from build123d import *

# Parameters (mm, degrees)
SKETCH1_W                = 20
SKETCH1_H                = 8
SKETCH1_R                = 1.25
BOSS_EXTRUDE1_DEPTH      = 2
BOSS_EXTRUDE2_DEPTH      = 4
BOSS_EXTRUDE2_DEPTH_BACK = 2
SKETCH3_R                = 0.5
SKETCH3_R_2              = 1
SKETCH5_R                = 1.5875
CUT_EXTRUDE1_DEPTH       = 4
FILLET1_R                = 1


with BuildPart() as part:
    # Sketch1 → Boss-Extrude1 (new body)
    with BuildSketch(Plane(origin=(0, 0, 0), x_dir=(1, 0, 0), z_dir=(0, 1, 0))):
        with Locations((10, 4)):
            Rectangle(SKETCH1_W, SKETCH1_H)
        with Locations(Location((4, 4, 0), (0, 0, 270))):
            Circle(SKETCH1_R, mode=Mode.SUBTRACT)
        with Locations(Location((16, 4, 0), (0, 0, 270))):
            Circle(SKETCH1_R, mode=Mode.SUBTRACT)
    extrude(amount=BOSS_EXTRUDE1_DEPTH)

    # Sketch3 → Boss-Extrude2 (add, two sides: drawn at the far end of the back side and taken through both)
    with BuildSketch(Plane.XY.offset(-BOSS_EXTRUDE2_DEPTH_BACK)):
        with BuildLine():
            Line((5.825, 2), (5.825, 6))
            ThreePointArc((5.825, 6), (10, 10.175), (14.175, 6))
            Line((14.175, 6), (14.175, 2))
            Line((14.175, 2), (14.175, 0))
            Line((14.175, 0), (5.825, 0))
            Line((5.825, 0), (5.825, 2))
        make_face()
        with Locations((10, 8.4875)):
            Circle(SKETCH3_R, mode=Mode.SUBTRACT)
        with Locations((12.154238192, 4.75625)):
            Circle(SKETCH3_R, mode=Mode.SUBTRACT)
        with Locations((7.845761808, 4.75625)):
            Circle(SKETCH3_R, mode=Mode.SUBTRACT)
        with Locations((10, 6)):
            Circle(SKETCH3_R_2, mode=Mode.SUBTRACT)
    extrude(amount=BOSS_EXTRUDE2_DEPTH + BOSS_EXTRUDE2_DEPTH_BACK)

    # Sketch5 → Cut-Extrude1 (cut)
    with BuildSketch(Plane.XY.offset(4)):
        with Locations((10, 6)):
            Circle(SKETCH5_R)
    extrude(amount=-CUT_EXTRUDE1_DEPTH, mode=Mode.SUBTRACT)

    # Fillet1
    fillet1_edges = [part.edges().sort_by_distance(p)[0] for p in [
        (10, 2, -2),
        (14.175, 2, -1),
        (5.825, 2, -1),
        (10, 0, 4),
    ]]
    fillet(fillet1_edges, radius=FILLET1_R)


solid = part.part
Work out the finished part from the listing and answer in its coordinate system (mm). A direction names the side the tool comes from. Give positions to 0.01 mm unless a question says otherwise; leave off trailing zeros. Loops run counter-clockwise (first coordinate to the right, second up) from the corner with the lowest first, then second, coordinate; pieces in that order, holes last. Notation, with made-up numbers: (86.25, 69.25) - (90.25, 69.25) arc R24 cw to (90.25, 94.25) - close; hole circle Ø1 at (84, 61). An arc over 180 degrees is marked (long way). Answer in a Markdown table with one row per item.
(1) Section C-C (y = 1.75) is taken. Give the vertices of the cut face in (x, z) (3 decimals).
Results list:
| item | result |
|---|---|
| outline | (0, -8) - (20, -8) - (20, 0) - (14.175, 0) - (14.175, 4) - (5.825, 4) - (5.825, 0) - (0, 0) - close; hole circle Ø2.5 at (4, -4); hole circle Ø2.5 at (16, -4) |
(2) A tool of negligible diameter and unlimited length cuts with its end or side. For faces 1 (the face through (3, 1, 0)), 2 (the face through (14.175, 3, 2)), 3 (the face through (5.825, 3, 2)), 4 (the face through (10, 4, 4)), from which of +Z, -Z, +X, -X, +Y, -Y can it reach the whole face along a straight path? Write none if from no direction.
Results list:
| item | result |
|---|---|
| face 1 | +Z, -X, +Y, -Y |
| face 2 | +Z, +X, +Y |
| face 3 | +Z, -X, +Y |
| face 4 | +Z, +X, -X, +Y, -Y |
(3) Flat-ended cylindrical pins translate along their axes: pin 1 Ø1 at (y, z) = (3.5, -2) entering from +X (3 decimals); pin 2 Ø1 at (x, z) = (13.5, -5.5) entering from +Y; pin 3 Ø1 at (x, y) = (9.5, 6.5) entering from +Z. Find the tip coordinate at first contact, or state that the pin passes through.
Results list:
| item | result |
|---|---|
| pin 1 | stops at x = 14.175 |
| pin 2 | stops at y = 2 |
| pin 3 | stops at z = 0 |
(4) Consider L1, parallel to X at y = 0.7, z = -4; L2, parallel to Y at x = 10, z = -0.65 (1 decimal); L3, parallel to X at y = 6, z = -0.45 (3 decimals). Determine where each line is inside the solid, lowest interval first. Write a range as [from, to].
Results list:
| item | result |
|---|---|
| L1 | x = [0, 2.75], [5.25, 14.75], [17.25, 20] |
| L2 | y = [0, 5], [7, 8], [9, 10.2] |
| L3 | x = [5.825, 9], [11, 14.175] |
(5) Section D-D (x = 10) is taken. Give the vertices of the cut face in (y, z) (1 decimal).
Results list:
| item | result |
|---|---|
| outline | (0, -8) - (2, -8) - (2, -3) arc R1 cw to (3, -2) - (5, -2) - (5, 0) - (4.4, 0) - (4.4, 4) - (1, 4) arc R1 ccw to (0, 3) - close; (7, -2) - (8, -2) - (8, 4) - (7.6, 4) - (7.6, 0) - (7, 0) - close; (9, -2) - (10.2, -2) - (10.2, 4) - (9, 4) - close |
(6) Section B-B (z = -4) is taken. Give the vertices of the cut face in (x, y), and give its area (3 significant figures).
Results list:
| item | result |
|---|---|
| outline | (0, 0) - (2.75, 0) - (2.75, 2) - (0, 2) - close; (5.25, 0) - (14.75, 0) - (14.75, 2) - (5.25, 2) - close; (17.25, 0) - (20, 0) - (20, 2) - (17.25, 2) - close |
| area | 30.0 mm² |
(7) Section A-A (x = 4) is taken. Give the vertices of the cut face in (y, z), and give its area (3 significant figures).
Results list:
| item | result |
|---|---|
| outline | (0, -8) - (2, -8) - (2, -5.25) - (0, -5.25) - close; (0, -2.75) - (2, -2.75) - (2, 0) - (0, 0) - close |
| area | 11.0 mm² |
(8) For a pull along X with two mould halves and no side action, classify faces 5 (the face through (5.54, 2.3, -1.15)), 6 (the face through (11, 7, -2)), 7 (the face through (7.346, 4.778, 0.958)), 8 (the face through (9, 7, 0)) as pulls with the +X half, pulls with the -X half, needs draft (parallel to the pull), parting line crosses it, or undercut.
Results list:
| item | result |
|---|---|
| face 5 | pulls with the -X half |
| face 6 | needs draft |
| face 7 | undercut |
| face 8 | undercut |
